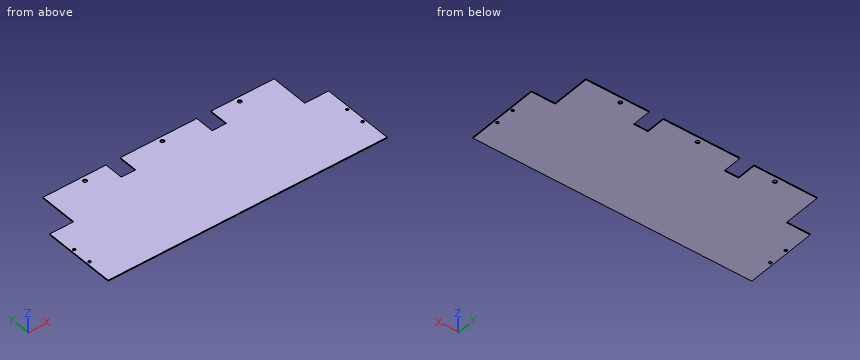
from build123d import *

# Parameters (mm, degrees)
SKETCH_1_R          = 1.5
EXTRUDE_1_DEPTH     = 1
SKETCH_2_R          = 2
SKETCH_2_W          = 15
SKETCH_2_H          = 20
CUT_EXTRUDE_1_DEPTH = 315.198981539


with BuildPart() as part:
    # 草图1 → 凸台-拉伸1 (new body)
    with BuildSketch(Plane.XY):
        Polygon((0, 0), (0, 76), (25, 76), (25, 116), (267, 116), (267, 76), (292, 76), (292, 0), align=None)
        with Locations((3, 48)):
            Circle(SKETCH_1_R, mode=Mode.SUBTRACT)
        with Locations((3, 28)):
            Circle(SKETCH_1_R, mode=Mode.SUBTRACT)
        with Locations(Location((289, 28, 0), (0, 0, 180))):
            Circle(SKETCH_1_R, mode=Mode.SUBTRACT)
        with Locations(Location((289, 48, 0), (0, 0, 180))):
            Circle(SKETCH_1_R, mode=Mode.SUBTRACT)
    extrude(amount=EXTRUDE_1_DEPTH)

    # 草图2 → 切除-拉伸1 (cut, through all)
    with BuildSketch(Plane.XY.offset(1)):
        with Locations((65, 111)):
            Circle(SKETCH_2_R)
        with Locations(Location((227, 111, 0), (0, 0, 180))):
            Circle(SKETCH_2_R)
        with Locations((146, 111)):
            Circle(SKETCH_2_R)
        with Locations((193.5, 106)):
            Rectangle(SKETCH_2_W, SKETCH_2_H)
        with Locations((98.5, 106)):
            Rectangle(SKETCH_2_W, SKETCH_2_H)
    extrude(amount=-CUT_EXTRUDE_1_DEPTH, mode=Mode.SUBTRACT)


solid = part.part
The model under review builds one solid part; all positions refer to its coordinate system, in mm. Give positions to 0.01 mm unless a question says otherwise; leave off trailing zeros. Order: outer loops, then holes, each group sorted by start corner. A loop starts at its lowest first (then second) coordinate and runs counter-clockwise, first axis right, second up. Notation, with made-up numbers: M 65,7.5 L 92,7.5 A20 ccw 92,29.5 Z; hole C 54.25,47 d2. An arc over 180 degrees is marked long. One line per question, with ' | ' between items. Start each with the question number.
1) Consider section A-A, the plane y = 105.5. Give the boundary of the cut face in (x, z), then the cut area to 3 significant figures.
2) Wall thickness on L1, parallel to Y at x = 289, z = 0.7; L2, parallel to Y at x = 227, z = 0.65; L3, parallel to X at y = 77.5, z = 0.8: over which ranges is each line inside the solid? List them lowest first. Write a range as from..to.
3) Clearance check with flat-ended pins moving along their axes: P1, Ø2.5, axis at x = 65, y = 111, coming from the -Z side; P2, Ø0.5, axis at y = 101.5, z = 0.5, coming from the -X side; P3, Ø0.5, axis at y = 108, z = 0.5, coming from the +X side. State where each tip first meets the part, or that it passes through.
4) Consider section B-B, the plane z = 0.45. Give the boundary of the cut face in (x, y), then the cut area to 3 significant figures.
5) Consider section C-C, the plane x = 271. Give the boundary of the cut face in (y, z), then the cut area to 3 significant figures.
Found:
1) outline: M 25,0 L 91,0 L 91,1 L 25,1 Z; M 106,0 L 186,0 L 186,1 L 106,1 Z; M 201,0 L 267,0 L 267,1 L 201,1 Z | area: 212 mm²
2) L1: y = 0..26.5, 29.5..46.5, 49.5..76 | L2: y = 0..109, 113..116 | L3: x = 25..267
3) P1: passes through | P2: stops at x = 25 | P3: stops at x = 267
4) outline: M 0,0 L 292,0 L 292,76 L 267,76 L 267,116 L 201,116 L 201,96 L 186,96 L 186,116 L 106,116 L 106,96 L 91,96 L 91,116 L 25,116 L 25,76 L 0,76 Z; hole C 3,28 d3; hole C 3,48 d3; hole C 65,111 d4; hole C 146,111 d4; hole C 227,111 d4; hole C 289,28 d3; hole C 289,48 d3 | area: 31,200 mm²
5) outline: M 0,0 L 76,0 L 76,1 L 0,1 Z | area: 76.0 mm²
